The model under review builds one solid part; all positions refer to its coordinate system, in mm. A direction names the side the tool comes from. Coordinates: 2 decimals unless noted, no trailing zeros. Write each loop counter-clockwise with the first axis right and the second up, starting at its lowest first coordinate (ties: lowest second). Pieces come first, ordered by that corner, then holes.
1) Add section B-B, the plane x = -25. State the section outline as (y, z) points, then the cut area to 3 significant figures.
2) Add section C-C, the plane y = -2. State the section outline as (x, z) points (1 decimal).
3) For P1, Ø1, axis at y = -10.5, z = 4.5, coming from the +X side; P2, Ø1.5, axis at y = -42, z = 15, coming from the -X side; P3, Ø16.5, axis at x = 34.5, z = 18.5, coming from the +Y side; P4, Ø10, axis at x = -12, y = -42, coming from the -Z side, all flat-tipped, find the tip position at first contact; note any pin that passes through.
4) For line 1 (X direction, y = -18.5, z = 3); line 2 (X direction, y = -33, z = 4); line 3 (Z direction, x = 4.5, y = -19.5), list the stretches that pass through material, from the lowest coordinate up.
5) Machinability: for faces 4 (the cylindrical face through (-35.928, -24.65, -31.438)), 5 (the cylindrical face through (33.951, -24.65, -31.447)), 6 (the cylindrical face through (34.01, -24.65, 29.22)), 7 (the cylindrical face through (37.078, -18.65, -27.586)), which of the approach directions +Z, -Z, +X, -X, +Y, -Y give a long, thin tool a straight path to every point of the face, cutting with its end or side? Answer none if there is none.
6) Add section D-D, the plane z = 15.5. State the section outline as (x, y) points.
7) Mouldability with a two-part tool opening along X and no side actions: class faces 1 (the flat face through (17, -44, 20)), 2 (the cylindrical face through (-37.06, 3.042, 36.128)), 3 (the cylindrical face through (54.21, 2.96, -27.33)) as released by +X, released by -X, zero draft, split by the parting line, or undercut.
8) Add section A-A, the plane y = -45.5. State the section outline as (x, z) points (1 decimal), then the cut area to 3 significant figures.
from build123d import *

# Parameters (mm, degrees)
BOSS_EXTRUDE1_DEPTH = 6
FILLET1_R           = 20
SKETCH4_W           = 3
SKETCH4_H           = 50
SKETCH6_R           = 16.245672788
CUT_EXTRUDE1_DEPTH  = 10
BOSS_EXTRUDE2_DEPTH = 3
CUT_EXTRUDE2_DEPTH  = 44
BOSS_EXTRUDE3_DEPTH = 53
SKETCH11_R          = 27.5
SKETCH11_R_2        = 7.5
CUT_EXTRUDE4_DEPTH  = 50


with BuildPart() as part:
    # Sketch1 → Boss-Extrude1 (new body)
    with BuildSketch(Plane(origin=(0, 0, 0), x_dir=(1, 0, 0), z_dir=(0, 1, 0))):
        with BuildLine():
            Line((34.540516942, 38.609131748), (-36.459483058, 38.609131748))
            ThreePointArc((-36.459483058, 38.609131748), (-66.459483058, 1.109131748), (-36.459483058, -36.390868252))
            Line((-36.459483058, -36.390868252), (34.540516942, -36.390868252))
            ThreePointArc((34.540516942, -36.390868252), (64.540516942, 1.109131748), (34.540516942, 38.609131748))
        make_face()
    extrude(amount=BOSS_EXTRUDE1_DEPTH)

    # Fillet1
    fillet1_edges = [part.edges().sort_by_distance(p)[0] for p in [
        (-36.459483058, 3, -38.609131748),
        (34.540516942, 3, -38.609131748),
        (34.540516942, 3, 36.390868252),
        (-36.459483058, 3, 36.390868252),
    ]]
    fillet(fillet1_edges, radius=FILLET1_R)

    # Sweep1: sweep along a path in Sketch3
    with BuildLine(Plane.XZ) as sweep1_path:
        Line((31.907446823, 29.390868252), (-33.82641294, 29.390868252))
        ThreePointArc((-33.82641294, 29.390868252), (-35.899239553, 29.224550102), (-37.919027907, 28.729851303))
        ThreePointArc((-37.919027907, 28.729851303), (-59.459483058, -1.109131748), (-37.919027907, -30.948114799))
        ThreePointArc((-37.919027907, -30.948114799), (-35.899239553, -31.442813598), (-33.82641294, -31.609131748))
        Line((-33.82641294, -31.609131748), (31.907446823, -31.609131748))
        ThreePointArc((31.907446823, -31.609131748), (33.980273437, -31.442813598), (36.000061791, -30.948114799))
        ThreePointArc((36.000061791, -30.948114799), (57.540516942, -1.109131748), (36.000061791, 28.729851303))
        ThreePointArc((36.000061791, 28.729851303), (33.980273437, 29.224550102), (31.907446823, 29.390868252))
    # Sketch4 → Sweep1 (sweep)
    with BuildSketch(Plane(origin=(31.907446823, 0, -31.609131748), x_dir=(0, 0, -1), z_dir=(1, 0, 0))):
        with Locations((-1.5, -25)):
            Rectangle(SKETCH4_W, SKETCH4_H)
    sweep(path=sweep1_path.line)

    # Sketch6 → Cut-Extrude1 (cut)
    with BuildSketch(Plane(origin=(0, 0, 0), x_dir=(1, 0, 0), z_dir=(0, 1, 0))):
        with Locations((75, 0)):
            Circle(SKETCH6_R)
        with Locations((-76.918966117, 0)):
            Circle(SKETCH6_R)
    extrude(amount=CUT_EXTRUDE1_DEPTH, mode=Mode.SUBTRACT)

    # Sketch7 → Boss-Extrude2 (add)
    with BuildSketch(Plane.XZ.offset(50)):
        with BuildLine():
            Line((31.907446823, 26.390868252), (-33.82641294, 26.390868252))
            ThreePointArc((-33.82641294, 26.390868252), (-35.42089495, 26.262931214), (-36.974578299, 25.882393676))
            ThreePointArc((-36.974578299, 25.882393676), (-56.459483058, -1.109131748), (-36.974578299, -28.100657171))
            ThreePointArc((-36.974578299, -28.100657171), (-35.42089495, -28.481194709), (-33.82641294, -28.609131748))
            Line((-33.82641294, -28.609131748), (31.907446823, -28.609131748))
            ThreePointArc((31.907446823, -28.609131748), (33.501928834, -28.481194709), (35.055612183, -28.100657171))
            ThreePointArc((35.055612183, -28.100657171), (54.540516942, -1.109131748), (35.055612183, 25.882393676))
            ThreePointArc((35.055612183, 25.882393676), (33.501928834, 26.262931214), (31.907446823, 26.390868252))
        make_face()
    extrude(amount=-BOSS_EXTRUDE2_DEPTH)

    # Sketch9 → Cut-Extrude2 (cut)
    with BuildSketch(Plane.XZ):
        with BuildLine():
            Line((-33.82641294, -28.609131748), (31.907446823, -28.609131748))
            ThreePointArc((31.907446823, -28.609131748), (33.501928834, -28.481194709), (35.055612183, -28.100657171))
            ThreePointArc((35.055612183, -28.100657171), (54.540516942, -1.109131748), (35.055612183, 25.882393676))
            ThreePointArc((35.055612183, 25.882393676), (33.501928834, 26.262931214), (31.907446823, 26.390868252))
            Line((31.907446823, 26.390868252), (-33.82641294, 26.390868252))
            ThreePointArc((-33.82641294, 26.390868252), (-35.42089495, 26.262931214), (-36.974578299, 25.882393676))
            ThreePointArc((-36.974578299, 25.882393676), (-56.459483058, -1.109131748), (-36.974578299, -28.100657171))
            ThreePointArc((-36.974578299, -28.100657171), (-35.42089495, -28.481194709), (-33.82641294, -28.609131748))
        make_face()
    extrude(amount=-CUT_EXTRUDE2_DEPTH, mode=Mode.SUBTRACT)

    # Sketch10 → Boss-Extrude3 (add)
    with BuildSketch(Plane(origin=(0, -47, 0), x_dir=(1, 0, 0), z_dir=(0, 1, 0))):
        with BuildLine():
            Line((31.907446823, 28.609131748), (-33.82641294, 28.609131748))
            ThreePointArc((-33.82641294, 28.609131748), (-35.42089495, 28.481194709), (-36.974578299, 28.100657171))
            ThreePointArc((-36.974578299, 28.100657171), (-56.459483058, 1.109131748), (-36.974578299, -25.882393676))
            ThreePointArc((-36.974578299, -25.882393676), (-35.42089495, -26.262931214), (-33.82641294, -26.390868252))
            Line((-33.82641294, -26.390868252), (31.907446823, -26.390868252))
            ThreePointArc((31.907446823, -26.390868252), (33.501928834, -26.262931214), (35.055612183, -25.882393676))
            ThreePointArc((35.055612183, -25.882393676), (54.540516942, 1.109131748), (35.055612183, 28.100657171))
            ThreePointArc((35.055612183, 28.100657171), (33.501928834, 28.481194709), (31.907446823, 28.609131748))
        make_face()
    extrude(amount=BOSS_EXTRUDE3_DEPTH)

    # Sketch11 → Cut-Extrude4 (cut)
    with BuildSketch(Plane(origin=(0, 6, 0), x_dir=(1, 0, 0), z_dir=(0, 1, 0))):
        with Locations(Location((-25, 0, 0), (0, 0, 270))):
            Circle(SKETCH11_R)
        with Locations(Location((16.748195248, 0.093303674, 0), (0, 0, 270))):
            Circle(SKETCH11_R_2)
        with Locations(Location((16.748195248, -19.906696326, 0), (0, 0, 270))):
            Circle(SKETCH11_R_2)
        with Locations(Location((16.486268254, 20.091588457, 0), (0, 0, 90))):
            Circle(SKETCH11_R_2)
        with Locations(Location((36.748195248, 0.093303674, 0), (0, 0, 270))):
            Circle(SKETCH11_R_2)
        with Locations(Location((36.748195248, -19.906696326, 0), (0, 0, 270))):
            Circle(SKETCH11_R_2)
        with Locations(Location((36.748195248, 20.093303674, 0), (0, 0, 270))):
            Circle(SKETCH11_R_2)
    extrude(amount=-CUT_EXTRUDE4_DEPTH, mode=Mode.SUBTRACT)


solid = part.part
Geometry results:
1. outline: (-50, -31.61) - (0, -31.61) - (0, -38.61) - (6, -38.61) - (6, -27.5) - (-44, -27.5) - (-44, 27.5) - (6, 27.5) - (6, 36.39) - (0, 36.39) - (0, 29.39) - (-50, 29.39) - close
1. area: 750 mm2
2. outline: (-37.9, -30.9) arc R13 ccw to (-33.8, -31.6) - (31.9, -31.6) arc R13 ccw to (36, -30.9) arc R31.4 ccw to (36, 28.7) arc R13 ccw to (31.9, 29.4) - (-33.8, 29.4) arc R13 ccw to (-37.9, 28.7) arc R31.4 ccw to start; hole circle Ø55 at (-25, 0); hole circle Ø15 at (16.5, -20.1); hole circle Ø15 at (16.7, -0.1); hole circle Ø15 at (16.7, 19.9); hole circle Ø15 at (36.7, -20.1); hole circle Ø15 at (36.7, -0.1); hole circle Ø15 at (36.7, 19.9)
3. P1: stops at x = 57.12
3. P2: stops at x = -55.45
3. P3: stops at y = 6
3. P4: stops at z = -31.61
4. line 1: x = -59.19 to -52.34, 2.34 to 9.92, 23.58 to 29.92, 43.58 to 57.27
4. line 2: x = -59.04 to -52.21, 2.21 to 10.46, 23.03 to 30.46, 43.03 to 57.12
4. line 3: z = -31.61 to 29.39
5. face 4: -Z, -X, -Y
5. face 5: -Z, +X, -Y
5. face 6: +Z, +X, -Y
5. face 7: +Y
6. outline: (-62.69, 0) - (-54.71, 0) - (-54.71, -50) - (52.79, -50) - (52.79, 0) - (60.77, 0) - (60.77, 6) - (42.82, 6) - (42.82, -44) - (30.68, -44) - (30.68, 6) - (22.82, 6) - (22.82, -44) - (10.68, -44) - (10.68, 6) - (-2.28, 6) - (-2.28, -44) - (-47.72, -44) - (-47.72, 6) - (-62.69, 6) - close
7. face 1: undercut
7. face 2: released by -X
7. face 3: released by +X
8. outline: (-37.9, -30.9) arc R13 ccw to (-33.8, -31.6) - (31.9, -31.6) arc R13 ccw to (36, -30.9) arc R31.4 ccw to (36, 28.7) arc R13 ccw to (31.9, 29.4) - (-33.8, 29.4) arc R13 ccw to (-37.9, 28.7) arc R31.4 ccw to start
8. area: 6,390 mm2
